Source: three-view drawing plus pictorial views. Frame: mm from the lowest corner of the part. Give positions to 0.01 mm unless a question says otherwise; leave off trailing zeros. Order: outer loops, then holes, each group sorted by start corner. A loop starts at its lowest first (then second) coordinate and runs counter-clockwise, first axis right, second up. Notation, with made-up numbers: M -21,28 L 13,28 A11 ccw 13,32 Z; hole C 45.25,68.5 d2. An arc over 180 degrees is marked long. Use CSV: the item, a comma, the result in double quotes. Start each with the question number.
Item 1: First-contact query: pin 1 (6 mm diameter, centred on y = 105.5, z = 19.5, fed in from -X); pin 2 (10 mm diameter, centred on y = 77, z = 37, fed in from -X) (3 decimals); pin 3 (6 mm diameter, centred on x = 31, y = 116.5, fed in from +Z); pin 4 (3 mm diameter, centred on x = 8, z = 42, fed in from -Y). Flat tips, straight axial feed; report the tip coordinate or a pass-through.
Item 2: Ray query, probe 1 along Y at (x, z) = (43.5, 35.5); probe 2 along X at (y, z) = (79, 20); probe 3 along Z at (x, y) = (27, 121.5). Return the intervals inside material, ascending. Write a range as from..to.
Item 3: Section query D-D on y = 73.5. Return loops of the section in (x, z), and give its area (3 significant figures).
Item 4: Section query B-B on x = 3. Return loops of the section in (y, z).
Item 5: Section query C-C on x = 25. Return loops of the section in (y, z), and give its area (3 significant figures).
Item 6: Section query A-A on z = 25. Return loops of the section in (x, y).
Item 7: Pull-direction query (Y, two-part tool) for the marked faces 1, 2, 3 and 4; classes: +Y half, -Y half, draft (parallel to the pull), parting line (faces both ways), or undercut.
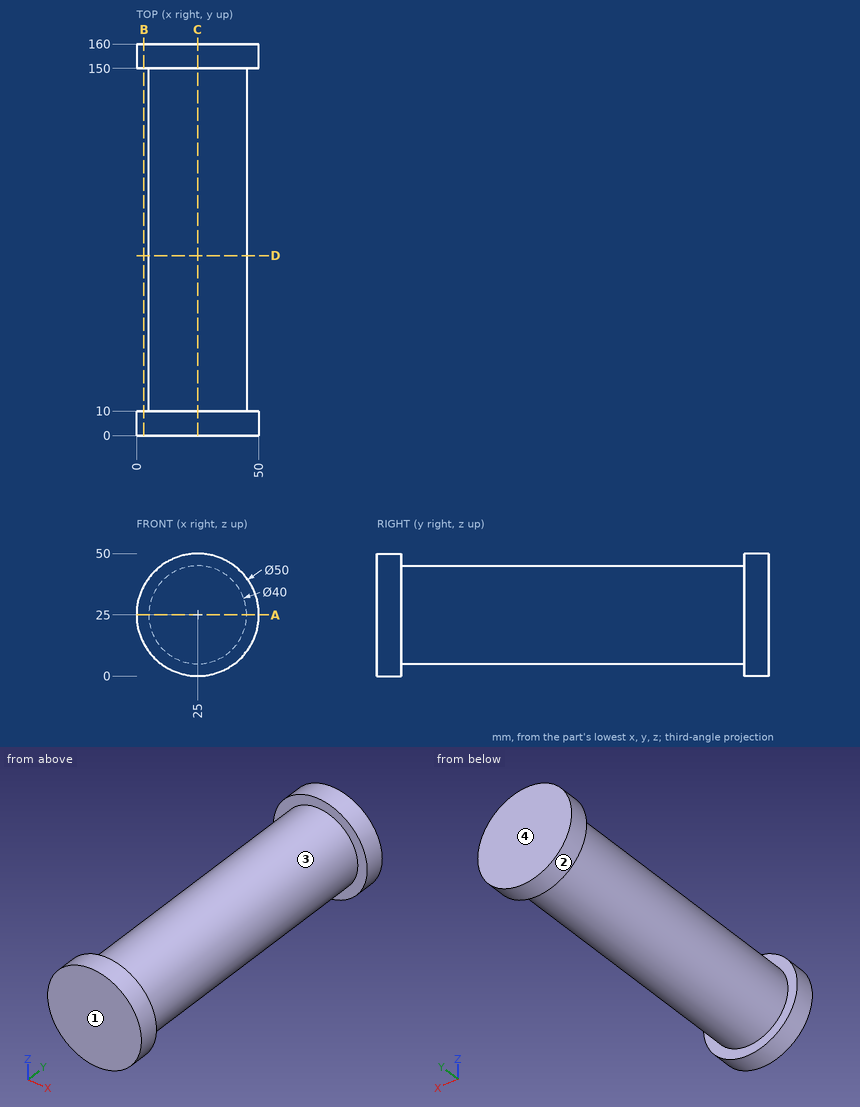
Verdict:
1,pin 1,"x = 5.16"
1,pin 2,"x = 6.265"
1,pin 3,"z = 44.77"
1,pin 4,"y = 0"
2,probe 1,"0..10, 150..160"
2,probe 2,"5.64..44.36"
2,probe 3,"5.1..44.9"
3,outline,"C 25,25 d40"
3,area,"1,260 mm2"
4,outline,"M 0,13.13 L 10,13.13 L 10,36.87 L 0,36.87 Z; M 150,13.13 L 160,13.13 L 160,36.87 L 150,36.87 Z"
5,outline,"M 0,0 L 10,0 L 10,5 L 150,5 L 150,0 L 160,0 L 160,50 L 150,50 L 150,45 L 10,45 L 10,50 L 0,50 Z"
5,area,"6,600 mm2"
6,outline,"M 0,0 L 50,0 L 50,10 L 45,10 L 45,150 L 50,150 L 50,160 L 0,160 L 0,150 L 5,150 L 5,10 L 0,10 Z"
7,face 1,"-Y half"
7,face 2,"draft"
7,face 3,"undercut"
7,face 4,"+Y half"
